Check sheet for the modelled part. Datum: model origin and axes. Units: mm. Face numbers are marked on the shaded views. Give positions to 0.01 mm unless a question says otherwise; leave off trailing zeros. Loops run counter-clockwise (first coordinate to the right, second up) from the corner with the lowest first, then second, coordinate; pieces in that order, holes last. Notation, with made-up numbers: (41, -3.75) - (69, -3.75) arc R26 ccw to (69, 30.25) - close; hole circle Ø2 at (35.5, -20). An arc over 180 degrees is marked (long way). Answer in a Markdown table with one row per item. Add a question column.
(1) Go/stop test with flat-tipped pins: P1, Ø6, axis at x = 1, y = -0.5, coming from the +Z side; P2, Ø5, axis at x = 0, y = 11.75, coming from the -Z side; P3, Ø4, axis at y = 7, z = 7.5, coming from the +X side; P4, Ø3, axis at y = 12, z = 2, coming from the -X side. Record where each tip stops, or that it passes through.
(2) Sectioned sample at D-D on x = 0. Enter the section's corners in (y, z).
(3) Draft check along Y on the marked faces 1, 2, 3 and 4. Enter one of: released by +Y, released by -Y, zero draft, split by the parting line, or undercut.
(4) Sectioned sample at A-A on z = 5. Enter the section's corners in (x, y), then the cut area to 3 significant figures.
(5) Sectioned sample at B-B on y = 11.75. Enter the section's corners in (x, z), then the cut area to 3 significant figures.
(6) Thickness scan on L1, parallel to Y at x = 0, z = 7.25; L2, parallel to Y at x = -2.5, z = 7; L3, parallel to Y at x = -0.5, z = 2.25. Record the ranges inside material, lowest first.
(7) Sectioned sample at C-C on z = 18.25. Enter the section's corners in (x, y), then the cut area to 3 significant figures.
from build123d import *

# Parameters (mm, degrees)
SKETCH1_R           = 21
BOSS_EXTRUDE1_DEPTH = 20
CUT_EXTRUDE1_DEPTH  = 17
CUT_EXTRUDE2_START  = -3
SKETCH3_R           = 4.25
CUT_EXTRUDE2_DEPTH  = 18


with BuildPart() as part:
    # Sketch1 → Boss-Extrude1 (new body)
    with BuildSketch(Plane.XY):
        Circle(SKETCH1_R)
    extrude(amount=BOSS_EXTRUDE1_DEPTH)

    # Sketch2 → Cut-Extrude1 (cut)
    with BuildSketch(Plane.XY.offset(20)):
        with BuildLine():
            Line((-2.75, 0), (0.522727273, 2.699862255))
            ThreePointArc((0.522727273, 2.699862255), (1.75, -2.121320344), (-2.75, 0))
        make_face()
    extrude(amount=-CUT_EXTRUDE1_DEPTH, mode=Mode.SUBTRACT)

    # Sketch3 → Cut-Extrude2 (cut)
    with BuildSketch(Plane.XY.offset(20).offset(CUT_EXTRUDE2_START)):
        with Locations((0, 11.75)):
            Circle(SKETCH3_R)
    extrude(amount=-CUT_EXTRUDE2_DEPTH, mode=Mode.SUBTRACT)


solid = part.part
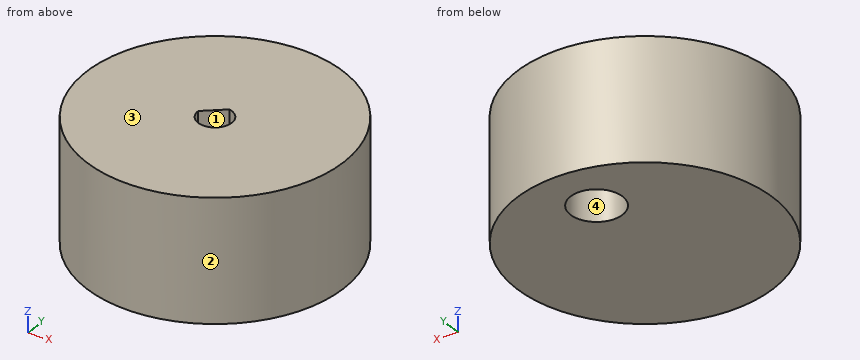
Reply:
| question | item | result |
|---|---|---|
| 1 | P1 | z = 20 |
| 1 | P2 | z = 17 |
| 1 | P3 | x = 20.4 |
| 1 | P4 | x = -18.19 |
| 2 | outline | (-21, 0) - (7.5, 0) - (7.5, 17) - (16, 17) - (16, 0) - (21, 0) - (21, 20) - (2.27, 20) - (2.27, 3) - (-2.75, 3) - (-2.75, 20) - (-21, 20) - close |
| 3 | face 1 | undercut |
| 3 | face 2 | split by the parting line |
| 3 | face 3 | zero draft |
| 3 | face 4 | undercut |
| 4 | outline | circle Ø42 at (0, 0); hole circle Ø8.5 at (0, 11.75); hole (-2.75, 0) arc R2.75 ccw (long way) to (0.52, 2.7) - close |
| 4 | area | 1,310 mm^2 |
| 5 | outline | (-17.41, 0) - (-4.25, 0) - (-4.25, 17) - (4.25, 17) - (4.25, 0) - (17.41, 0) - (17.41, 20) - (-17.41, 20) - close |
| 5 | area | 552 mm^2 |
| 6 | L1 | -21 to -2.75, 2.27 to 7.5, 16 to 21 |
| 6 | L2 | -20.85 to -1.15, 0.21 to 8.31, 15.19 to 20.85 |
| 6 | L3 | -20.99 to 7.53, 15.97 to 20.99 |
| 7 | outline | circle Ø42 at (0, 0); hole (-2.75, 0) arc R2.75 ccw (long way) to (0.52, 2.7) - close |
| 7 | area | 1,360 mm^2 |
